Input: part model. Units: mm. Frame: model coordinates. A direction names the side the tool comes from. Round coordinates to 2 decimals unless told otherwise and drop trailing zeros. Loops run counter-clockwise (first coordinate to the right, second up) from the corner with the lowest first, then second, coordinate; pieces in that order, holes last. Notation, with made-up numbers: M 53,68.5 L 75,68.5 A10 ccw 75,73.5 Z; hole C -12.5,-12.75 d3. An arc over 180 degrees is marked long. Use one line per item in the form item = value. Start each with the question number.
Q1. Ray query, line 1 along X through (y, z) = (6.9, 0); line 2 along X through (y, z) = (0.3, 0); line 3 along X through (y, z) = (4.5, 0). Return the intervals inside material, ascending.
Q2. Section query C-C, the plane y = 4.75. Output: boundary loops of the cut face in (x, z).
Q3. Mould query, pull axis X, two halves, no side actions, for faces 1 (the flat face through (-6, 6.5, 2)), 2 (the flat face through (9, 7, -3)), 3 (the cylindrical face through (3.755, 6.24, 11.923)). Classes: pulls with the +X half, pulls with the -X half, needs draft (parallel to the pull), parting line crosses it, or undercut.
Q4. Access query for faces 4 (the flat face through (-9, 0, 2)), 5 (the cylindrical face through (1.802, 6.754, 5.723)), 6 (the cylindrical face through (-2.703, 0.254, 8.584)). Directions: +Z, -Z, +X, -X, +Y, -Y. A direction counts if a zero-diameter tool reaches every point of the face in a straight line with its end or side. Return the directions, or none.
Q5. Section query A-A, the plane x = 0. Output: boundary loops of the cut face in (y, z), and give its area (3 significant figures).
Q6. Section query D-D, the plane z = -6.5. Output: boundary loops of the cut face in (x, y), and give its area (3 significant figures).
Q7. Section query B-B, the plane z = 0. Output: boundary loops of the cut face in (x, y).
```python
from build123d import *

# Parameters (mm, degrees)
SKETCH1_R           = 11
SKETCH1_R_2         = 4
BOSS_EXTRUDE1_DEPTH = 5.5
SKETCH2_R           = 12.5
SKETCH2_R_2         = 4
BOSS_EXTRUDE2_DEPTH = 1.5
SKETCH3_R           = 9
SKETCH3_R_2         = 6
CUT_EXTRUDE1_DEPTH  = 0.5
CUT_EXTRUDE2_START  = -0.5
SKETCH4_R           = 9
SKETCH4_R_2         = 6
CUT_EXTRUDE2_DEPTH  = 0.5


with BuildPart() as part:
    # Sketch1 → Boss-Extrude1 (new body)
    with BuildSketch(Plane(origin=(0, 0, 0), x_dir=(1, 0, 0), z_dir=(0, 1, 0))):
        with Locations(Location((0, 0, 0), (0, 0, 270))):
            Circle(SKETCH1_R)
        with Locations(Location((0, 0, 0), (0, 0, 270))):
            Circle(SKETCH1_R_2, mode=Mode.SUBTRACT)
    extrude(amount=BOSS_EXTRUDE1_DEPTH)

    # Sketch2 → Boss-Extrude2 (add)
    with BuildSketch(Plane(origin=(0, 5.5, 0), x_dir=(1, 0, 0), z_dir=(0, 1, 0))):
        with Locations(Location((0, 0, 0), (0, 0, 270))):
            Circle(SKETCH2_R)
        with Locations(Location((0, 0, 0), (0, 0, 270))):
            Circle(SKETCH2_R_2, mode=Mode.SUBTRACT)
    extrude(amount=BOSS_EXTRUDE2_DEPTH)

    # Sketch3 → Cut-Extrude1 (cut)
    with BuildSketch(Plane(origin=(0, 7, 0), x_dir=(1, 0, 0), z_dir=(0, 1, 0))):
        with Locations(Location((0, 0, 0), (0, 0, 270))):
            Circle(SKETCH3_R)
        with Locations(Location((0, 0, 0), (0, 0, 270))):
            Circle(SKETCH3_R_2, mode=Mode.SUBTRACT)
    extrude(amount=-CUT_EXTRUDE1_DEPTH, mode=Mode.SUBTRACT)

    # Sketch4 → Cut-Extrude2 (cut)
    with BuildSketch(Plane.XZ.offset(CUT_EXTRUDE2_START)):
        with Locations(Location((0, 0, 0), (0, 0, 90))):
            Circle(SKETCH4_R)
        with Locations(Location((0, 0, 0), (0, 0, 90))):
            Circle(SKETCH4_R_2, mode=Mode.SUBTRACT)
    extrude(amount=CUT_EXTRUDE2_DEPTH, mode=Mode.SUBTRACT)


solid = part.part
```
Results found:
q1.line_1 = -12.5 to -9, -6 to -4, 4 to 6, 9 to 12.5
q1.line_2 = -11 to -9, -6 to -4, 4 to 6, 9 to 11
q1.line_3 = -11 to -4, 4 to 11
q2.outline = C 0,0 d22; hole C 0,0 d8
q3.face_1 = undercut
q3.face_2 = needs draft
q3.face_3 = parting line crosses it
q4.face_4 = +Z, -Z, +X, -X, -Y
q4.face_5 = +Y
q4.face_6 = -Y
q5.outline = M 0,-11 L 5.5,-11 L 5.5,-12.5 L 7,-12.5 L 7,-9 L 6.5,-9 L 6.5,-6 L 7,-6 L 7,-4 L 0,-4 L 0,-6 L 0.5,-6 L 0.5,-9 L 0,-9 Z; M 0,4 L 7,4 L 7,6 L 6.5,6 L 6.5,9 L 7,9 L 7,12.5 L 5.5,12.5 L 5.5,11 L 0,11 L 0,9 L 0.5,9 L 0.5,6 L 0,6 Z
q5.area = 96.5 mm²
q6.outline = M -10.68,5.5 L -8.87,5.5 L -8.87,0 L -6.22,0 L -6.22,0.5 L 6.22,0.5 L 6.22,0 L 8.87,0 L 8.87,5.5 L 10.68,5.5 L 10.68,7 L 6.22,7 L 6.22,6.5 L -6.22,6.5 L -6.22,7 L -10.68,7 Z
q6.area = 117 mm²
q7.outline = M -12.5,5.5 L -11,5.5 L -11,0 L -9,0 L -9,0.5 L -6,0.5 L -6,0 L -4,0 L -4,7 L -6,7 L -6,6.5 L -9,6.5 L -9,7 L -12.5,7 Z; M 4,0 L 6,0 L 6,0.5 L 9,0.5 L 9,0 L 11,0 L 11,5.5 L 12.5,5.5 L 12.5,7 L 9,7 L 9,6.5 L 6,6.5 L 6,7 L 4,7 Z
